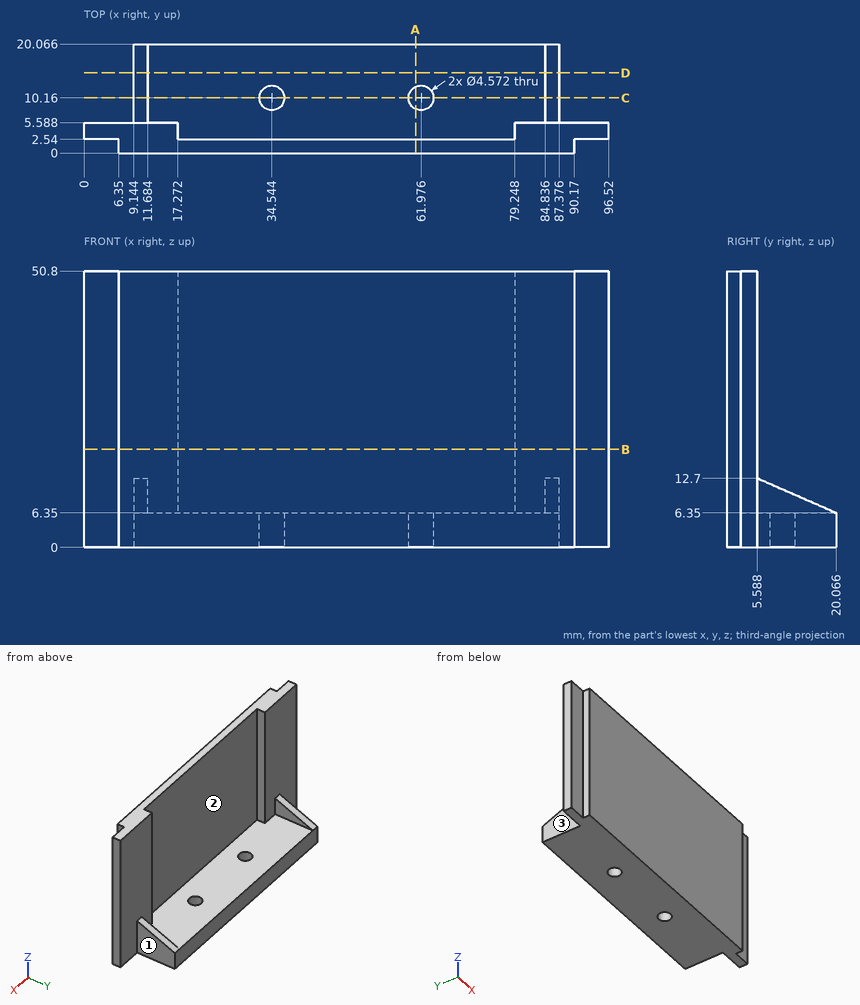
Check sheet for the drawn part. Datum: minimum x, y, z corner. Units: mm. Round coordinates to 2 decimals unless told otherwise and drop trailing zeros. Order: outer loops, then holes, each group sorted by start corner. A loop starts at its lowest first (then second) coordinate and runs counter-clockwise, first axis right, second up.
1. Section check B-B on z = 18. Record the cut outline in (x, y).
Final values:
outline: (0, 2.54) - (6.35, 2.54) - (6.35, 0) - (90.17, 0) - (90.17, 2.54) - (96.52, 2.54) - (96.52, 5.59) - (79.25, 5.59) - (79.25, 2.54) - (17.27, 2.54) - (17.27, 5.59) - (0, 5.59) - close
2. Section check D-D on y = 14.75. Record the cut outline in (x, z), then the cut area to 3 significant figures.
Final values:
outline: (9.14, 0) - (87.38, 0) - (87.38, 8.68) - (84.84, 8.68) - (84.84, 6.35) - (11.68, 6.35) - (11.68, 8.68) - (9.14, 8.68) - close
area: 509 mm2
3. Thickness scan on L1, parallel to Y at x = 47.5, z = 20.5; L2, parallel to Y at x = 4.5, z = 19.5; L3, parallel to Z at x = 58.5, y = 14.25. Record the ranges inside material, lowest first.
Final values:
L1: y = 0 to 2.54
L2: y = 2.54 to 5.59
L3: z = 0 to 6.35
4. Section check C-C on y = 10.16. Record the cut outline in (x, z).
Final values:
outline: (9.14, 0) - (32.26, 0) - (32.26, 6.35) - (11.68, 6.35) - (11.68, 10.69) - (9.14, 10.69) - close; (36.83, 0) - (59.69, 0) - (59.69, 6.35) - (36.83, 6.35) - close; (64.26, 0) - (87.38, 0) - (87.38, 10.69) - (84.84, 10.69) - (84.84, 6.35) - (64.26, 6.35) - close
5. Go/stop test with flat-tipped pins: P1, Ø1.9, axis at x = 2, z = 23, coming from the -Y side; P2, Ø5.5, axis at x = 61.976, y = 10.16, coming from the +Z side; P3, Ø1.5, axis at x = 63.5, z = 40, coming from the +Y side. Record where each tip stops, or that it passes through.
Final values:
P1: stops at y = 2.54
P2: stops at z = 6.35
P3: stops at y = 2.54
6. Section check A-A on x = 61. Record the cut outline in (y, z).
Final values:
outline: (0, 0) - (8.09, 0) - (8.09, 6.35) - (2.54, 6.35) - (2.54, 50.8) - (0, 50.8) - close; (12.23, 0) - (20.07, 0) - (20.07, 6.35) - (12.23, 6.35) - close
7. Release check for a two-part mould opening along X. For the marked faces 1, 2 and 3 record: +X half, -X half, draft (parallel to the pull), parting line (faces both ways), or undercut.
Final values:
face 1: +X half
face 2: undercut
face 3: -X half
